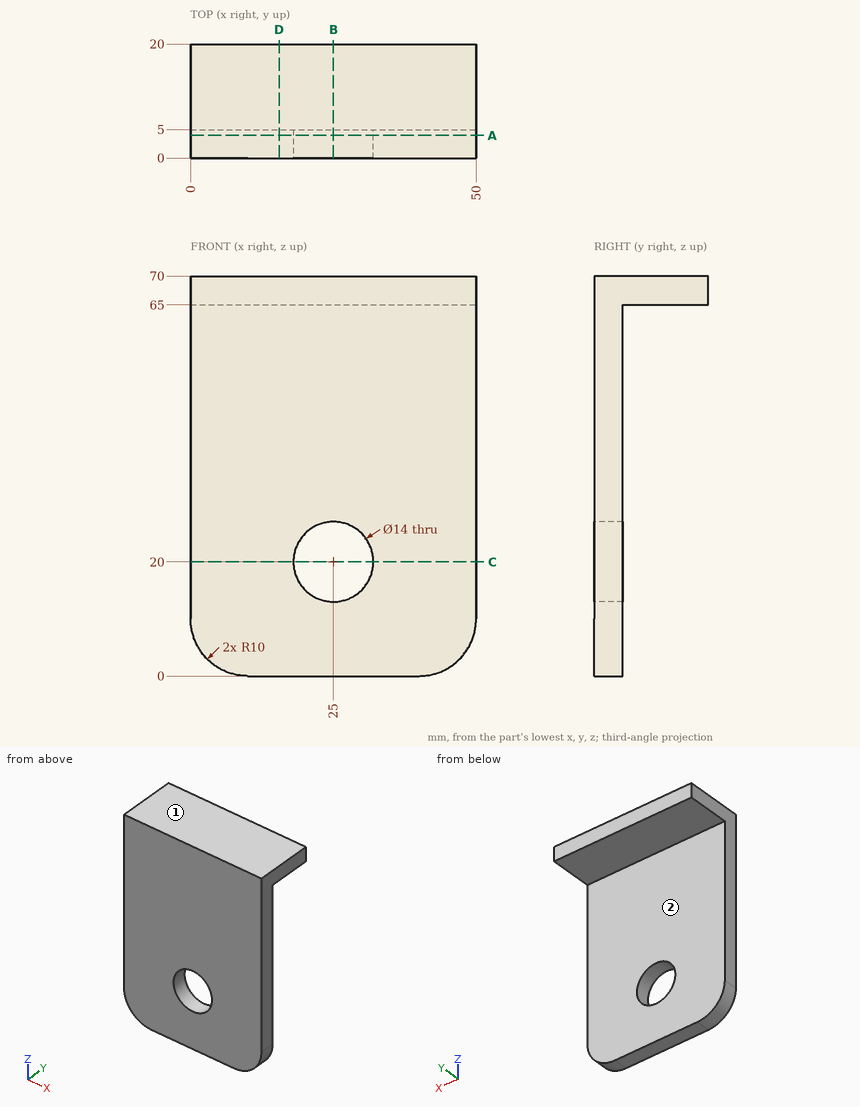
Could you check a few things on this drawing? It's one solid part, dimensions in mm from its lowest x, y, z. A direction names the side the tool comes from. Give positions to 0.01 mm unless a question says otherwise; leave off trailing zeros. Order: outer loops, then holes, each group sorted by start corner. A loop starts at its lowest first (then second) coordinate and runs counter-clockwise, first axis right, second up. Notation, with made-up numbers: (53, 76.25) - (95, 76.25) arc R28 ccw to (95, 101.25) - close; hole circle Ø3 at (20, -37). An arc over 180 degrees is marked (long way). One line per question, with ' | ' between items. Start each with the question number.
Item 1: For the marked faces 1 and 2, which set-ups out of +Z, -Z, +X, -X, +Y, -Y let a thin tool reach every point of the face, with its end or its side?
Item 2: I need wall thicknesses on probe 1 along Y at (x, z) = (20.5, 47); probe 2 along Z at (x, y) = (25, 2.65); probe 3 along Z at (x, y) = (10, 14.5). Which ranges of each line are inside material? Lowest first, please. Write a range as [from, to].
Item 3: I'm going to push flat-ended pins straight in: pin 1 Ø2 at (y, z) = (7, 40.5) entering from +X; pin 2 Ø25 at (x, z) = (35, 40) entering from +Y; pin 3 Ø1.5 at (x, y) = (25, 12) entering from -Z. Where does each tip first touch, or does it pass through?
Item 4: I want a section at C-C on z = 20. Write out the boundary of the cut face in (x, y).
Item 5: I want a section at A-A on y = 4. Write out the boundary of the cut face in (x, z).
Item 6: I want a section at D-D on x = 15.5. Write out the boundary of the cut face in (y, z).
Item 7: I want a section at B-B on x = 25. Write out the boundary of the cut face in (y, z).
Verdict:
1) face 1: +Z, +X, -X, +Y, -Y | face 2: -Z, +X, -X, +Y
2) probe 1: [0, 5] | probe 2: [0, 13], [27, 70] | probe 3: [65, 70]
3) pin 1: through | pin 2: y = 5 | pin 3: z = 65
4) outline: (0, 0) - (18, 0) - (18, 5) - (0, 5) - close; (32, 0) - (50, 0) - (50, 5) - (32, 5) - close
5) outline: (0, 10) arc R10 ccw to (10, 0) - (40, 0) arc R10 ccw to (50, 10) - (50, 70) - (0, 70) - close; hole circle Ø14 at (25, 20)
6) outline: (0, 0) - (5, 0) - (5, 65) - (20, 65) - (20, 70) - (0, 70) - close
7) outline: (0, 0) - (5, 0) - (5, 13) - (0, 13) - close; (0, 27) - (5, 27) - (5, 65) - (20, 65) - (20, 70) - (0, 70) - close
